Read the model definition and answer for the solid it produces. Units are mm, in the model's axes. Face numbers are marked on the shaded views. A direction names the side the tool comes from. Coordinates: 2 decimals unless noted, no trailing zeros. Loops run counter-clockwise (first coordinate to the right, second up) from the corner with the lowest first, then second, coordinate; pieces in that order, holes last. Notation, with made-up numbers: (6.5, 73) -> (65.5, 73) arc R15 ccw to (65.5, 86) -> close; hole circle Ø9 at (75.5, 7.5). An arc over 180 degrees is marked (long way). Answer as a JSON object with one key per item and string values. Group by question number.
1) Section C-C, the plane y = -45 is taken. Give the vertices of the cut face in (x, z).
2) Flat-ended cylindrical pins translate along their axes: P1, Ø12.5, axis at y = -113.5, z = -7.5, coming from the +X side; P2, Ø1.5, axis at y = -126.5, z = 16, coming from the -X side; P3, Ø11, axis at x = 42.5, y = -81, coming from the +Z side; P4, Ø3, axis at x = 29, z = -18.5, coming from the -Y side. Find the tip coordinate at first contact, or state that the pin passes through.
3) Section B-B, the plane z = -13.5 is taken. Give the vertices of the cut face in (x, y).
4) Determine the mould class of the marked faces 1, 2, 3 and 4 for opening direction X: released by +X, released by -X, zero draft, split by the parting line, or undercut.
5) Section D-D, the plane x = 0 is taken. Give the vertices of the cut face in (y, z), plus the area to 3 significant figures.
6) Section A-A, the plane y = -127 is taken. Give the vertices of the cut face in (x, z).
7) Which of the six approach directions +Z, -Z, +X, -X, +Y, -Y give full straight-line access (tool end or side, diameter ignored) to the marked faces 5, 6, 7 and 8?
8) Consider probe 1 along X at (y, z) = (-142, -2.5); probe 2 along X at (y, z) = (-49.5, 1.5); probe 3 along Z at (x, y) = (-48.5, -80). Determine where each line is inside the solid, lowest interval first. Write a range as [from, to].
from build123d import *

# Parameters (mm, degrees)
BOSS_EXTRUDE1_DEPTH = 152.4
SKETCH2_R           = 4.7625
CUT_EXTRUDE1_DEPTH  = 50.8
FILLET1_R           = 6.35
SKETCH3_W           = 22.225
SKETCH3_H           = 4.7625
CUT_EXTRUDE3_DEPTH  = 2.651


with BuildPart() as part:
    # Sketch1 → Boss-Extrude1 (new body)
    with BuildSketch(Plane(origin=(0, 0, 0), x_dir=(1, 0, 0), z_dir=(0, 1, 0))):
        with BuildLine():
            Line((-27.051, 0), (-27.051, 23.749))
            Line((-27.051, 23.749), (-63.5, 23.749))
            Line((-63.5, 23.749), (-63.5, 25.4))
            Line((-63.5, 25.4), (-25.4, 25.4))
            Line((-25.4, 25.4), (-25.4, 0))
            ThreePointArc((-25.4, 0), (0, -25.4), (25.4, 0))
            Line((25.4, 0), (25.4, 25.4))
            Line((25.4, 25.4), (63.5, 25.4))
            Line((63.5, 25.4), (63.5, 23.749))
            Line((63.5, 23.749), (27.051, 23.749))
            Line((27.051, 23.749), (27.051, 0))
            ThreePointArc((27.051, 0), (0, -27.051), (-27.051, 0))
        make_face()
    extrude(amount=-BOSS_EXTRUDE1_DEPTH)

    # Sketch2 → Cut-Extrude1 (cut)
    with BuildSketch(Plane.XY.offset(-23.749)):
        with Locations((-45.2755, -25.4)):
            Circle(SKETCH2_R)
        with Locations((45.2755, -25.4)):
            Circle(SKETCH2_R)
        with Locations((-45.2755, -127)):
            Circle(SKETCH2_R)
        with Locations((45.2755, -127)):
            Circle(SKETCH2_R)
    extrude(amount=-CUT_EXTRUDE1_DEPTH, mode=Mode.SUBTRACT)

    # Fillet1
    fillet1_edges = [part.edges().sort_by_distance(p)[0] for p in [
        (63.5, 0, -24.5745),
        (-63.5, 0, -24.5745),
        (-63.5, -152.4, -24.5745),
        (63.5, -152.4, -24.5745),
    ]]
    fillet(fillet1_edges, radius=FILLET1_R)

    # Sketch3 → Cut-Extrude3 (cut, through all)
    with BuildSketch(Plane.XY.offset(-23.749)):
        with Locations((45.2755, -114.3)):
            Rectangle(SKETCH3_W, SKETCH3_H)
        with Locations((-45.2755, -114.3)):
            Rectangle(SKETCH3_W, SKETCH3_H)
    extrude(amount=-CUT_EXTRUDE3_DEPTH, mode=Mode.SUBTRACT)


solid = part.part
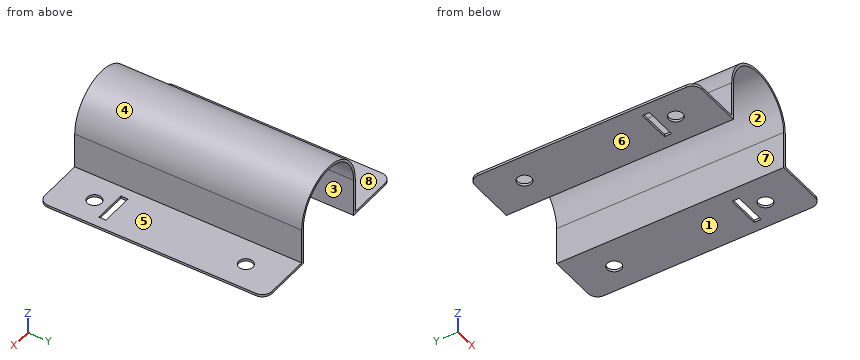
Determined:
{
 "1": {"outline": "(-63.5, -25.4) -> (-25.4, -25.4) -> (-25.4, 0) arc R25.4 cw to (25.4, 0) -> (25.4, -25.4) -> (63.5, -25.4) -> (63.5, -23.75) -> (27.05, -23.75) -> (27.05, 0) arc R27.05 ccw to (-27.05, 0) -> (-27.05, -23.75) -> (-63.5, -23.75) -> close"},
 "2": {"P1": "x = 27.05", "P2": "x = -22.34", "P3": "z = -23.75", "P4": "through"},
 "3": {"outline": "(-27.05, -152.4) -> (-25.4, -152.4) -> (-25.4, 0) -> (-27.05, 0) -> close; (25.4, -152.4) -> (27.05, -152.4) -> (27.05, 0) -> (25.4, 0) -> close"},
 "4": {"face 1": "zero draft", "face 2": "undercut", "face 3": "undercut", "face 4": "split by the parting line"},
 "5": {"outline": "(-152.4, 25.4) -> (0, 25.4) -> (0, 27.05) -> (-152.4, 27.05) -> close", "area": "252 mm²"},
 "6": {"outline": "(-63.5, -25.4) -> (-50.04, -25.4) -> (-50.04, -23.75) -> (-63.5, -23.75) -> close; (-40.51, -25.4) -> (-25.4, -25.4) -> (-25.4, 0) arc R25.4 cw to (25.4, 0) -> (25.4, -25.4) -> (40.51, -25.4) -> (40.51, -23.75) -> (27.05, -23.75) -> (27.05, 0) arc R27.05 ccw to (-27.05, 0) -> (-27.05, -23.75) -> (-40.51, -23.75) -> close; (50.04, -25.4) -> (63.5, -25.4) -> (63.5, -23.75) -> (50.04, -23.75) -> close"},
 "7": {"face 5": "+Z, +X, +Y, -Y", "face 6": "-Z, +X, -X, +Y, -Y", "face 7": "-Z, +Y, -Y", "face 8": "+Z, -X, +Y, -Y"},
 "8": {"probe 1": "[-27.05, -25.4], [25.4, 27.05]", "probe 2": "[-27.01, -25.36], [25.36, 27.01]", "probe 3": "[-25.4, -23.75]"}
}
